```python
from build123d import *

# Parameters (mm, degrees)
CROQUIS1_W              = 40
CROQUIS1_H              = 50
SALIENTE_EXTRUIR1_DEPTH = 5
CROQUIS2_W              = 20
CROQUIS2_H              = 50
SALIENTE_EXTRUIR2_DEPTH = 40
CORTAR_EXTRUIR1_REACH   = 72.178
REDONDEO1_R             = 2
CORTAR_EXTRUIR2_REACH   = 57.227
CROQUIS4_R              = 3.175
REDONDEO2_R             = 3


with BuildPart() as part:
    # Croquis1 → Saliente-Extruir1 (new body)
    with BuildSketch(Plane.XY):
        Rectangle(CROQUIS1_W, CROQUIS1_H)
    extrude(amount=SALIENTE_EXTRUIR1_DEPTH)

    # Croquis2 → Saliente-Extruir2 (add)
    with BuildSketch(Plane.XY.offset(5)):
        Rectangle(CROQUIS2_W, CROQUIS2_H)
    extrude(amount=SALIENTE_EXTRUIR2_DEPTH)

    # Croquis3 → Cortar-Extruir1 (cut, up to next)
    with BuildSketch(Plane(origin=(0, 25, 0), x_dir=(1, 0, 0), z_dir=(0, 1, 0)), mode=Mode.PRIVATE) as cortar_extruir1_sk1:
        Polygon((-6, 0), (-3.5, -10), (3.5, -10), (6, 0), align=None)
    cortar_extruir1_tool1 = extrude(cortar_extruir1_sk1.sketch, amount=-CORTAR_EXTRUIR1_REACH, mode=Mode.PRIVATE) & part.part
    add(cortar_extruir1_tool1.solids().sort_by_distance((0, 25, 4.561404))[0], mode=Mode.SUBTRACT)

    # Redondeo1
    redondeo1_edges = [part.edges().sort_by_distance(p)[0] for p in [
        (-6, 0, 0),
        (6, 0, 0),
    ]]
    fillet(redondeo1_edges, radius=REDONDEO1_R)

    # Croquis4 → Cortar-Extruir2 (cut, up to next)
    with BuildSketch(Plane.XY.offset(45), mode=Mode.PRIVATE) as cortar_extruir2_sk1:
        Circle(CROQUIS4_R)
    cortar_extruir2_tool1 = extrude(cortar_extruir2_sk1.sketch, amount=-CORTAR_EXTRUIR2_REACH, mode=Mode.PRIVATE) & part.part
    add(cortar_extruir2_tool1.solids().sort_by_distance((0, 0, 45))[0], mode=Mode.SUBTRACT)

    # Redondeo2
    redondeo2_edges = [part.edges().sort_by_distance(p)[0] for p in [
        (10, 0, 45),
        (-10, 0, 45),
    ]]
    fillet(redondeo2_edges, radius=REDONDEO2_R)


solid = part.part
```
Can you work these out from the model? Positions are in its coordinate system, mm. A direction names the side the tool comes from. Coordinates: 2 decimals unless noted, no trailing zeros. Loops run counter-clockwise (first coordinate to the right, second up) from the corner with the lowest first, then second, coordinate; pieces in that order, holes last.
1) Imagine slicing it at C-C on z = 34.5. List the corners of the cut face in (x, y) for me (3 decimals).
2) Imagine slicing it at B-B on y = 0. List the corners of the cut face in (x, z) for me (3 decimals), plus the area to 3 significant figures.
3) Imagine slicing it at A-A on x = 0. List the corners of the cut face in (y, z) for me (3 decimals).
4) Thinking about a two-plate mould opening in X: for faces 5 (the flat face through (4.546, 0.35, 5.817)), 6 (the flat face through (14, 0, 0)), 7 (the flat face through (-20, 0, 2)), 8 (the flat face through (20, 0, 2)), which applies, pulls with the +X half, pulls with the -X half, needs draft (parallel to the pull), parting line crosses it, or undercut?
5) For pin 1 (5 mm diameter, centred on y = -7, z = 21, fed in from -X); pin 2 (4 mm diameter, centred on x = 14, y = -1, fed in from +Z); pin 3 (8 mm diameter, centred on y = 14, z = 35.5, fed in from +X), each with a flat end and sliding along its axis, tell me the tip position at first contact or that it passes through.
6) Which directions (+Z, -Z, +X, -X, +Y, -Y) give clear straight access to the entire face, cutting with the end or side of a thin tool? Please do faces 1 (the flat face through (15, 0, 5)), 2 (the flat face through (-4.575, 0.35, 5.698)), 3 (the flat face through (-10, 0, 23)), 4 (the cylindrical face through (-0.69, -3.1, 27.74)).
7) I need wall thicknesses on probe 1 along Y at (x, z) = (0, 26.5) (3 decimals); probe 2 along Z at (x, y) = (-10.5, 20); probe 3 along X at (y, z) = (12.5, 24). Which ranges of each line are inside material? Lowest first, please.
8) Imagine slicing it at D-D on y = -12. List the corners of the cut face in (x, z) for me.
Completed:
1. outline: (-10, -25) - (10, -25) - (10, 25) - (-10, 25) - close; hole circle Ø6.35 at (0, 0)
2. outline: (-20, 0) - (-7.562, 0) arc R2 ccw to (-5.621, 1.515) - (-3.5, 10) - (-3.175, 10) - (-3.175, 45) - (-7, 45) arc R3 ccw to (-10, 42) - (-10, 5) - (-20, 5) - close; (3.175, 10) - (3.5, 10) - (5.621, 1.515) arc R2 ccw to (7.562, 0) - (20, 0) - (20, 5) - (10, 5) - (10, 42) arc R3 ccw to (7, 45) - (3.175, 45) - close
2. area: 678 mm2
3. outline: (-25, 10) - (-3.175, 10) - (-3.175, 45) - (-25, 45) - close; (3.175, 10) - (25, 10) - (25, 45) - (3.175, 45) - close
4. face 5: undercut
4. face 6: needs draft
4. face 7: pulls with the -X half
4. face 8: pulls with the +X half
5. pin 1: stops at x = -10
5. pin 2: stops at z = 5
5. pin 3: stops at x = 10
6. face 1: +Z, +X, +Y, -Y
6. face 2: -Z, +Y, -Y
6. face 3: +Z, -X, +Y, -Y
6. face 4: +Z, -Z
7. probe 1: y = -25 to -3.175, 3.175 to 25
7. probe 2: z = 0 to 5
7. probe 3: x = -10 to 10
8. outline: (-20, 0) - (-7.56, 0) arc R2 ccw to (-5.62, 1.51) - (-3.5, 10) - (3.5, 10) - (5.62, 1.51) arc R2 ccw to (7.56, 0) - (20, 0) - (20, 5) - (10, 5) - (10, 42) arc R3 ccw to (7, 45) - (-7, 45) arc R3 ccw to (-10, 42) - (-10, 5) - (-20, 5) - close
